```python
from build123d import *

# Parameters (mm, degrees)
SKETCH2_R               = 1.75
BOSS_EXTRUDE1_DEPTH     = 3
BOSS_EXTRUDE1_2_DEPTH   = 3
BOSS_EXTRUDE2_START     = -3
BOSS_EXTRUDE2_DEPTH     = 3
SKETCH5_W               = 3
SKETCH5_H               = 37.771572876
BOSS_EXTRUDE3_DEPTH     = 2
BOSS_EXTRUDE4_DEPTH     = 3
CUT_EXTRUDE1_DEPTH      = 10
SKETCH9_R               = 11.5
CUT_EXTRUDE2_DEPTH      = 10
FILL_PATTERN1_OUTLINE_R = 1.75
FILL_PATTERN1_DEPTH     = 3


# Read off the part's stored shape, not the designer's step: Fill Pattern1
with BuildPart() as part:
    # Sketch2 → Boss-Extrude1 (new body)
    with BuildSketch(Plane.XY):
        with BuildLine():
            Line((31.67162959, -17.664113805), (31.67162959, 9.835886195))
            Line((31.67162959, 9.835886195), (21.67162959, 19.835886195))
            Line((21.67162959, 19.835886195), (-22.32837041, 19.835886195))
            Line((-22.32837041, 19.835886195), (-32.32837041, 9.835886195))
            Line((-32.32837041, 9.835886195), (-32.32837041, -17.664113805))
            ThreePointArc((-32.32837041, -17.664113805), (-29.399438222, -24.735181617), (-22.32837041, -27.664113805))
            Line((-22.32837041, -27.664113805), (21.67162959, -27.664113805))
            ThreePointArc((21.67162959, -27.664113805), (28.742697402, -24.735181617), (31.67162959, -17.664113805))
        make_face()
        with Locations((18.67162959, 5.585886195)):
            Circle(SKETCH2_R, mode=Mode.SUBTRACT)
        with Locations((1.17162959, -13.314113805)):
            Circle(SKETCH2_R, mode=Mode.SUBTRACT)
        with Locations((-23.82837041, -3.214113805)):
            Circle(SKETCH2_R, mode=Mode.SUBTRACT)
        with Locations((-9.82837041, -3.214113805)):
            Circle(SKETCH2_R, mode=Mode.SUBTRACT)
    extrude(amount=BOSS_EXTRUDE1_DEPTH)



with BuildPart() as body_2:
    # Sketch2 → Boss-Extrude1 2 (new body)
    with BuildSketch(Plane.XY):
        with BuildLine():
            Line((-2.02837041, -32.69254093), (-2.02837041, -65.435686681))
            ThreePointArc((-2.02837041, -65.435686681), (-1.898965615, -66.086248516), (-1.530451938, -66.637768209))
            Line((-1.530451938, -66.637768209), (1.097975187, -69.266195333))
            ThreePointArc((1.097975187, -69.266195333), (1.64949488, -69.634709011), (2.300056715, -69.764113805))
            Line((2.300056715, -69.764113805), (35.043202465, -69.764113805))
            ThreePointArc((35.043202465, -69.764113805), (35.6937643, -69.634709011), (36.245283993, -69.266195333))
            Line((36.245283993, -69.266195333), (38.873711118, -66.637768209))
            ThreePointArc((38.873711118, -66.637768209), (39.242224795, -66.086248516), (39.37162959, -65.435686681))
            Line((39.37162959, -65.435686681), (39.37162959, -32.69254093))
            ThreePointArc((39.37162959, -32.69254093), (39.242224795, -32.041979095), (38.873711118, -31.490459402))
            Line((38.873711118, -31.490459402), (36.245283993, -28.862032277))
            ThreePointArc((36.245283993, -28.862032277), (35.6937643, -28.4935186), (35.043202465, -28.364113805))
            Line((35.043202465, -28.364113805), (2.300056715, -28.364113805))
            ThreePointArc((2.300056715, -28.364113805), (1.64949488, -28.4935186), (1.097975187, -28.862032277))
            Line((1.097975187, -28.862032277), (-1.530451938, -31.490459402))
            ThreePointArc((-1.530451938, -31.490459402), (-1.898965615, -32.041979095), (-2.02837041, -32.69254093))
        make_face()
        with Locations((34.17162959, -33.564113805)):
            Circle(SKETCH2_R, mode=Mode.SUBTRACT)
        with Locations((3.17162959, -33.564113805)):
            Circle(SKETCH2_R, mode=Mode.SUBTRACT)
        with Locations((34.17162959, -64.564113805)):
            Circle(SKETCH2_R, mode=Mode.SUBTRACT)
        with Locations((3.17162959, -64.564113805)):
            Circle(SKETCH2_R, mode=Mode.SUBTRACT)
    extrude(amount=BOSS_EXTRUDE1_2_DEPTH)


with BuildPart() as part_1:
    add(part.part)

    add(body_2.part)  # Boss-Extrude2 merges body 2
    # Sketch3 → Boss-Extrude2 (add)
    with BuildSketch(Plane.XY.offset(3).offset(BOSS_EXTRUDE2_START)):
        with BuildLine():
            Line((-2.02837041, -32.69254093), (-2.02837041, -27.664113805))
            Line((-2.02837041, -27.664113805), (21.67162959, -27.664113805))
            ThreePointArc((21.67162959, -27.664113805), (28.742697402, -24.735181617), (31.67162959, -17.664113805))
            Line((31.67162959, -17.664113805), (31.67162959, -8.484617852))
            Line((31.67162959, -8.484617852), (39.67162959, -20.545709175))
            Line((39.67162959, -20.545709175), (39.67162959, -32.69254093))
            Line((39.67162959, -32.69254093), (35.689147538, -32.69254093))
            ThreePointArc((35.689147538, -32.69254093), (34.17162959, -31.814113805), (32.654111642, -32.69254093))
            Line((32.654111642, -32.69254093), (4.689147538, -32.69254093))
            ThreePointArc((4.689147538, -32.69254093), (3.17162959, -31.814113805), (1.654111642, -32.69254093))
            Line((1.654111642, -32.69254093), (-2.02837041, -32.69254093))
        make_face()
    extrude(amount=BOSS_EXTRUDE2_DEPTH)

    # Sketch5 → Boss-Extrude3 (add)
    with BuildSketch(Plane.ZY.offset(2.02837041)):
        with Locations((1.5, -46.549900243)):
            Rectangle(SKETCH5_W, SKETCH5_H)
    extrude(amount=BOSS_EXTRUDE3_DEPTH)

    # Sketch6 → Boss-Extrude4 (add)
    with BuildSketch(Plane.ZY.offset(4.02837041)):
        Polygon((3, -27.664113805), (0, -27.664113805), (0, -65.435686681), (3, -65.435686681), (25, -43.435686681), (25, -13.435686681), (3, -5.428341527), align=None)
    extrude(amount=BOSS_EXTRUDE4_DEPTH)

    # Sketch7 → Cut-Extrude1 (cut)
    with BuildSketch(Plane.XY.offset(3)):
        Polygon((-24.32837041, -23.70556569), (-20.82837041, -21.684839748), (-20.82837041, -17.643387863), (-24.32837041, -15.622661921), (-27.82837041, -17.643387863), (-27.82837041, -21.684839748), align=None)
    extrude(amount=-CUT_EXTRUDE1_DEPTH, mode=Mode.SUBTRACT)

    # Sketch9 → Cut-Extrude2 (cut)
    with BuildSketch(Plane.XY.offset(3)):
        with Locations((18.67162959, -49.064113805)):
            Circle(SKETCH9_R)
    extrude(amount=-CUT_EXTRUDE2_DEPTH, mode=Mode.SUBTRACT)

    # Fill Pattern1 outline → Fill Pattern1 (cut)
    # profile 1 of 16: a face of its own
    with BuildSketch(Plane.XY):
        Polygon((13.812645741, 2.356612137), (10.312645741, 4.377338079), (6.812645741, 2.356612137), (6.812645741, -1.684839748), (10.312645741, -3.70556569), (13.812645741, -1.684839748), align=None)
    # profile 2 of 16: a face of its own
    with BuildSketch(Plane.XY):
        Polygon((22.472899779, 7.356612137), (18.972899779, 9.377338079), (15.472899779, 7.356612137), (15.472899779, 3.315160252), (18.972899779, 1.29443431), (22.472899779, 3.315160252), align=None)
        with Locations((18.67162959, 5.585886195)):
            Circle(FILL_PATTERN1_OUTLINE_R, mode=Mode.SUBTRACT)
    # profile 3 of 16: a face of its own
    with BuildSketch(Plane.XY):
        Polygon((-12.168116372, -12.643387863), (-15.668116372, -10.622661921), (-19.168116372, -12.643387863), (-19.168116372, -16.684839748), (-15.668116372, -18.70556569), (-12.168116372, -16.684839748), align=None)
    # profile 4 of 16: a face of its own
    with BuildSketch(Plane.XY):
        Polygon((6.812645741, -27.643387863), (6.812645741, -31.684839748), (10.312645741, -33.70556569), (13.812645741, -31.684839748), (13.812645741, -27.643387863), (10.312645741, -25.622661921), align=None)
    # profile 5 of 16: a face of its own
    with BuildSketch(Plane.XY):
        Polygon((10.312645741, 14.377338079), (6.812645741, 12.356612137), (6.812645741, 8.315160252), (10.312645741, 6.29443431), (13.812645741, 8.315160252), (13.812645741, 12.356612137), align=None)
    # profile 6 of 16: a face of its own
    with BuildSketch(Plane.XY):
        Polygon((10.312645741, -15.622661921), (6.812645741, -17.643387863), (6.812645741, -21.684839748), (10.312645741, -23.70556569), (13.812645741, -21.684839748), (13.812645741, -17.643387863), align=None)
    # profile 7 of 16: a face of its own
    with BuildSketch(Plane.XY):
        Polygon((10.312645741, -5.622661921), (6.812645741, -7.643387863), (6.812645741, -11.684839748), (10.312645741, -13.70556569), (13.812645741, -11.684839748), (13.812645741, -7.643387863), align=None)
    # profile 8 of 16: a face of its own
    with BuildSketch(Plane.XY):
        Polygon((22.472899779, -22.643387863), (18.972899779, -20.622661921), (15.472899779, -22.643387863), (15.472899779, -26.684839748), (18.972899779, -28.70556569), (22.472899779, -26.684839748), align=None)
    # profile 9 of 16: a face of its own
    with BuildSketch(Plane.XY):
        Polygon((31.133153817, -17.643387863), (27.633153817, -15.622661921), (24.133153817, -17.643387863), (24.133153817, -21.684839748), (27.633153817, -23.70556569), (31.133153817, -21.684839748), align=None)
    # profile 10 of 16: a face of its own
    with BuildSketch(Plane.XY):
        Polygon((-1.847608297, 7.356612137), (-1.847608297, 3.315160252), (1.652391703, 1.29443431), (5.152391703, 3.315160252), (5.152391703, 7.356612137), (1.652391703, 9.377338079), align=None)
    # profile 11 of 16: a face of its own
    with BuildSketch(Plane.XY):
        Polygon((15.472899779, -2.643387863), (15.472899779, -6.684839748), (18.972899779, -8.70556569), (22.472899779, -6.684839748), (22.472899779, -2.643387863), (18.972899779, -0.622661921), align=None)
    # profile 12 of 16: a face of its own
    with BuildSketch(Plane.XY):
        Polygon((-10.507862334, 12.356612137), (-10.507862334, 8.315160252), (-7.007862334, 6.29443431), (-3.507862334, 8.315160252), (-3.507862334, 12.356612137), (-7.007862334, 14.377338079), align=None)
    # profile 13 of 16: a face of its own
    with BuildSketch(Plane.XY):
        Polygon((-12.168116372, -2.643387863), (-15.668116372, -0.622661921), (-19.168116372, -2.643387863), (-19.168116372, -6.684839748), (-15.668116372, -8.70556569), (-12.168116372, -6.684839748), align=None)
    # profile 14 of 16: a face of its own
    with BuildSketch(Plane.XY):
        Polygon((18.972899779, -10.622661921), (15.472899779, -12.643387863), (15.472899779, -16.684839748), (18.972899779, -18.70556569), (22.472899779, -16.684839748), (22.472899779, -12.643387863), align=None)
    # profile 15 of 16: a face of its own
    with BuildSketch(Plane.XY):
        Polygon((-19.168116372, 7.356612137), (-19.168116372, 3.315160252), (-15.668116372, 1.29443431), (-12.168116372, 3.315160252), (-12.168116372, 7.356612137), (-15.668116372, 9.377338079), align=None)
    # profile 16 of 16: a face of its own
    with BuildSketch(Plane.XY):
        Polygon((24.133153817, -27.643387863), (24.133153817, -31.684839748), (27.633153817, -33.70556569), (31.133153817, -31.684839748), (31.133153817, -27.643387863), (27.633153817, -25.622661921), align=None)
    extrude(amount=FILL_PATTERN1_DEPTH, mode=Mode.SUBTRACT)


solid = part_1.part
```
Read the model definition and answer for the solid it produces. Units are mm, in the model's axes. A direction names the side the tool comes from. Coordinates: 2 decimals unless noted, no trailing zeros. Loops run counter-clockwise (first coordinate to the right, second up) from the corner with the lowest first, then second, coordinate; pieces in that order, holes last. Notation, with made-up numbers: (0.25, 17) -> (18.25, 17) arc R12 cw to (18.25, 40) -> close; hole circle Ø10 at (-29.75, 12). An arc over 180 degrees is marked (long way). Return JSON: item names as keys, results as strings.
Item 1: Find section D-D (y = -48). Determine the outline of the cut face in (x, z).
Answers:
{"outline": "(-7.03, 0) -> (7.22, 0) -> (7.22, 3) -> (-4.03, 3) -> (-4.03, 20.44) -> (-7.03, 20.44) -> close; (30.12, 0) -> (39.37, 0) -> (39.37, 3) -> (30.12, 3) -> close"}
Item 2: For a pull along Y with two mould halves and no side action, classify faces 1 (the flat face through (26.74, 14.77, 1.48)), 2 (the flat face through (-17.394, -1.619, 1.479)), 3 (the flat face through (31.672, 1, 1)) as +Y half, -Y half, draft (parallel to the pull), parting line (faces both ways), or undercut.
Answers:
{"face 1": "+Y half", "face 2": "undercut", "face 3": "draft"}
Item 3: Flat-ended cylindrical pins translate along their axes: P1, Ø10, axis at y = -42.5, z = 2.5, coming from the +X side; P2, Ø3, axis at x = -9.83, y = -3.21, coming from the +Z side; P3, Ø0.9, axis at y = -29, z = 2, coming from the -X side; P4, Ø1.5, axis at y = 6, z = 1.5, coming from the +X side. Find the tip coordinate at first contact, or state that the pin passes through.
Answers:
{"P1": "stops at x = 39.37", "P2": "passes through", "P3": "stops at x = -7.03", "P4": "stops at x = 31.67"}
Item 4: Find the intervals of material crossed by probe 1 along Y at (x, z) = (27, 2); probe 2 along X at (y, z) = (-53, 7.5); probe 3 along Z at (x, y) = (15, -3.5), in increasing order.
Answers:
{"probe 1": "y = -69.76 to -56.99, -41.13 to -33.34, -25.99 to -23.34, -15.99 to 14.51", "probe 2": "x = -7.03 to -4.03", "probe 3": "z = 0 to 3"}
Item 5: Find section B-B (x = 12). Determine the outline of the cut face in (y, z).
Answers:
{"outline": "(-69.76, 0) -> (-58.43, 0) -> (-58.43, 3) -> (-69.76, 3) -> close; (-39.7, 0) -> (-32.73, 0) -> (-32.73, 3) -> (-39.7, 3) -> close; (-26.6, 0) -> (-22.73, 0) -> (-22.73, 3) -> (-26.6, 3) -> close; (-16.6, 0) -> (-12.73, 0) -> (-12.73, 3) -> (-16.6, 3) -> close; (-6.6, 0) -> (-2.73, 0) -> (-2.73, 3) -> (-6.6, 3) -> close; (3.4, 0) -> (7.27, 0) -> (7.27, 3) -> (3.4, 3) -> close; (13.4, 0) -> (19.84, 0) -> (19.84, 3) -> (13.4, 3) -> close"}
Item 6: Find section C-C (x = -17.5). Determine the outline of the cut face in (y, z), plus the area to 3 significant figures.
Answers:
{"outline": "(-27.66, 0) -> (-17.65, 0) -> (-17.65, 3) -> (-27.66, 3) -> close; (-11.68, 0) -> (-7.65, 0) -> (-7.65, 3) -> (-11.68, 3) -> close; (-1.68, 0) -> (2.35, 0) -> (2.35, 3) -> (-1.68, 3) -> close; (8.32, 0) -> (19.84, 0) -> (19.84, 3) -> (8.32, 3) -> close", "area": "88.8 mm2"}
Item 7: For faces 4 (the flat face through (29.41, -16.65, 1.48)), 5 (the flat face through (-32.328, -4, 1)), 6 (the flat face through (-4.028, -35, 11)), determine the directions among +Z, -Z, +X, -X, +Y, -Y from which every point of the face is accessible in a straight line to the end or side of a thin tool.
Answers:
{"face 4": "+Z, -Z", "face 5": "+Z, -Z, -X, +Y, -Y", "face 6": "+Z, +X, +Y, -Y"}
Item 8: Find section A-A (y = -30). Determine the outline of the cut face in (x, z).
Answers:
{"outline": "(-7.03, 0) -> (6.81, 0) -> (6.81, 3) -> (-4.03, 3) -> (-4.03, 25) -> (-7.03, 25) -> close; (13.81, 0) -> (24.13, 0) -> (24.13, 3) -> (13.81, 3) -> close; (31.13, 0) -> (39.67, 0) -> (39.67, 3) -> (31.13, 3) -> close"}
